The model under review builds one solid part; all positions refer to its coordinate system, in mm. Round coordinates to 2 decimals unless told otherwise and drop trailing zeros. Order: outer loops, then holes, each group sorted by start corner. A loop starts at its lowest first (then second) coordinate and runs counter-clockwise, first axis right, second up. Notation, with made-up numbers: M 20,48 L 34,48 A27 cw 34,73 Z; hole C 83.25,58.25 d5. An arc over 180 degrees is marked long. One line per item, written item: value. Start each with the question number.
from build123d import *

# Parameters (mm, degrees)
LEG_START     = -10.839044341
LEG_OUTLINE_R = 2.65
LEG_DEPTH     = 6


# Read off the part's stored shape, not the designer's step: leg
with BuildPart() as part:
    # leg outline → leg (new body)
    with BuildSketch(Plane(origin=(0, 0, 0), x_dir=(1, 0, 0), z_dir=(0, 1, 0)).offset(LEG_START)):
        Polygon((-105.386140363, -62.9747167), (224.613859637, -62.9747167), (224.613859637, 71.5252833), (64.213859637, 71.5252833), (64.213859637, 65.5252833), (-1.886140363, 65.5252833), (-1.886140363, 392.5252833), (-31.886140363, 392.5252833), (-105.386140363, 71.5252833), align=None)
        with Locations((-53.636140363, -56.9747167)):
            Circle(LEG_OUTLINE_R, mode=Mode.SUBTRACT)
        with Locations((1.113859637, -29.3497167)):
            Circle(LEG_OUTLINE_R, mode=Mode.SUBTRACT)
        with Locations((59.238859637, -56.9747167)):
            Circle(LEG_OUTLINE_R, mode=Mode.SUBTRACT)
        with Locations((1.113859637, 37.9002833)):
            Circle(LEG_OUTLINE_R, mode=Mode.SUBTRACT)
        with BuildLine():
            Line((16.413859637, 26.8252833), (16.413859637, 36.3252833))
            ThreePointArc((16.413859637, 36.3252833), (17.292539294, 38.446603644), (19.413859637, 39.3252833))
            Line((19.413859637, 39.3252833), (48.813859637, 39.3252833))
            ThreePointArc((48.813859637, 39.3252833), (50.935179981, 38.446603644), (51.813859637, 36.3252833))
            Line((51.813859637, 36.3252833), (51.813859637, 26.8252833))
            ThreePointArc((51.813859637, 26.8252833), (50.93517998, 24.703962956), (48.813859637, 23.8252833))
            Line((48.813859637, 23.8252833), (19.413859637, 23.8252833))
            ThreePointArc((19.413859637, 23.8252833), (17.292539294, 24.703962957), (16.413859637, 26.8252833))
        make_face(mode=Mode.SUBTRACT)
        with Locations((169.488859637, -56.9747167)):
            Circle(LEG_OUTLINE_R, mode=Mode.SUBTRACT)
    extrude(amount=LEG_DEPTH)


solid = part.part
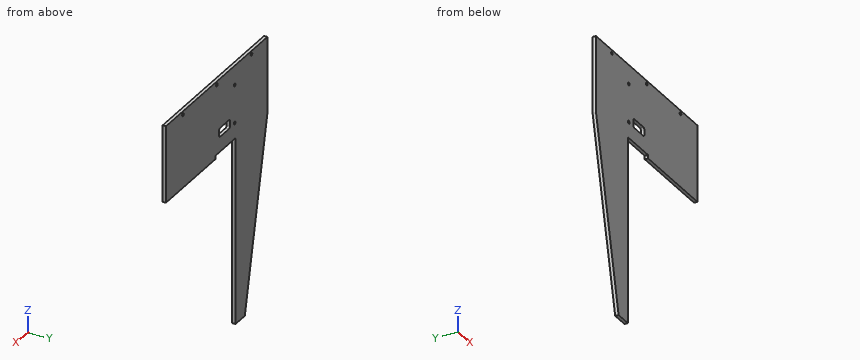
Item 1: Consider section A-A, the plane y = -6.3. Give the boundary of the cut face in (x, z), then the cut area to 3 significant figures.
Item 2: Consider section C-C, the plane z = -140.5. Give the boundary of the cut face in (x, y), then the cut area to 3 significant figures.
Item 3: Consider section B-B, the plane x = 110. Give the boundary of the cut face in (y, z).
Item 4: Clearance check with flat-ended pins moving along their axes: P1, Ø1.5, axis at x = 99.5, y = -9, coming from the -Z side; P2, Ø1.5, axis at y = -6.5, z = -229, coming from the +X side; P3, Ø3, axis at x = 1.11, z = -37.9, coming from the -Y side; P4, Ø1.8, axis at x = 37.5, y = -8, coming from the -Z side. State where each tip first meets the part, or that it passes through.
Item 5: Wall thickness on L1, parallel to Z at x = 45.5, y = -8.4; L2, parallel to Z at x = 58.5, y = -8.65; L3, parallel to X at y = -6.1, z = -35.5: over which ranges is each line inside the solid? List them lowest first.
Computed:
1. outline: M -105.39,-71.53 L -31.89,-392.53 L -1.89,-392.53 L -1.89,-65.53 L 64.21,-65.53 L 64.21,-71.53 L 224.61,-71.53 L 224.61,62.97 L -105.39,62.97 Z; hole C -53.64,56.97 d5.3; hole C 1.11,-37.9 d5.3; hole C 1.11,29.35 d5.3; hole M 16.41,-36.33 A3 ccw 19.41,-39.33 L 48.81,-39.33 A3 ccw 51.81,-36.33 L 51.81,-26.83 A3 ccw 48.81,-23.83 L 19.41,-23.83 A3 ccw 16.41,-26.83 Z; hole C 59.24,56.97 d5.3; hole C 169.49,56.97 d5.3
1. area: 64,800 mm^2
2. outline: M -89.59,-10.84 L -1.89,-10.84 L -1.89,-4.84 L -89.59,-4.84 Z
2. area: 526 mm^2
3. outline: M -10.84,-71.53 L -4.84,-71.53 L -4.84,62.97 L -10.84,62.97 Z
4. P1: stops at z = -71.53
4. P2: stops at x = -1.89
4. P3: passes through
4. P4: stops at z = -65.53
5. L1: z = -65.53 to -39.33, -23.83 to 62.97
5. L2: z = -65.53 to 54.43, 59.52 to 62.97
5. L3: x = -105.39 to -0.01, 2.24 to 16.41, 51.81 to 224.61
